Can you work these out from the model? Positions are in its coordinate system, mm. A direction names the side the tool comes from. Coordinates: 2 decimals unless noted, no trailing zeros. Loops run counter-clockwise (first coordinate to the right, second up) from the corner with the lowest first, then second, coordinate; pieces in that order, holes last.
```python
from build123d import *

# Parameters (mm, degrees)
BOSS_EXTRUDE1_DEPTH = 9
SKETCH2_R           = 1.2
CUT_EXTRUDE1_DEPTH  = 29


with BuildPart() as part:
    # Sketch1 → Boss-Extrude1 (new body)
    with BuildSketch(Plane.XY):
        Polygon((7.5, 1), (7.5, 11.5), (-7.5, 11.5), (-7.5, 1), (-11.5, 1), (-11.5, 0), (-6.5, 0), (-6.5, 10.5), (6.5, 10.5), (6.5, 0), (11.5, 0), (11.5, 1), align=None)
    extrude(amount=BOSS_EXTRUDE1_DEPTH)

    # Sketch2 → Cut-Extrude1 (cut)
    with BuildSketch(Plane(origin=(0, 1, 0), x_dir=(1, 0, 0), z_dir=(0, 1, 0))):
        with Locations((9.5, -4.5)):
            Circle(SKETCH2_R)
    cut_extrude1 = extrude(amount=-CUT_EXTRUDE1_DEPTH, mode=Mode.SUBTRACT)

    # Mirror1: Cut-Extrude1 across plane
    add(cut_extrude1.mirror(Plane(origin=(0, 0, 0), x_dir=(0, 0, 1), z_dir=(1, 0, 0))), mode=Mode.SUBTRACT)


solid = part.part
```
Item 1: I'm going to push flat-ended pins straight in: P1, Ø3, axis at x = -10, z = 6.5, coming from the +Y side; P2, Ø3, axis at x = -1, z = 7, coming from the -Y side; P3, Ø2.5, axis at y = 2.5, z = 6, coming from the -X side. Where does each tip first touch, or does it pass through?
Results are:
P1: stops at y = 1
P2: stops at y = 10.5
P3: stops at x = -7.5
Item 2: On a 3-axis mill with a long thin cutter (end or side, diameter ignored), from which of +Z, -Z, +X, -X, +Y, -Y can I reach the whole of each face in a straight line? I mean faces 4 (the face through (7.5, 6, 4)), 5 (the face through (-8.3, 0.51, 4.45)), 6 (the face through (-8, 0, 4)), 7 (the face through (-6.5, 5, 4)), 8 (the face through (-11, 1, 4)). Say none if no direction works.
Results are:
face 4: +Z, -Z, +X, +Y
face 5: +Y, -Y
face 6: +Z, -Z, +X, -X, -Y
face 7: +Z, -Z, -Y
face 8: +Z, -Z, -X, +Y
Item 3: Suppose I cut it at A-A, the plane x = 9.5. Please give me the cut outline in (y, z), plus the area to 3 significant figures.
Results are:
outline: (0, 0) - (1, 0) - (1, 3.3) - (0, 3.3) - close; (0, 5.7) - (1, 5.7) - (1, 9) - (0, 9) - close
area: 6.60 mm2
Item 4: Suppose I cut it at B-B, the plane y = 2. Please give me the cut outline in (x, z).
Results are:
outline: (-7.5, 0) - (-6.5, 0) - (-6.5, 9) - (-7.5, 9) - close; (6.5, 0) - (7.5, 0) - (7.5, 9) - (6.5, 9) - close
Item 5: I need wall thicknesses on line 1 along X through (y, z) = (0.5, 4.5); line 2 along Z through (x, y) = (9.5, 0.4); line 3 along X through (y, z) = (9.75, 1.5). Which ranges of each line are inside material? Lowest first, please.
Results are:
line 1: x = -11.5 to -10.7, -8.3 to -6.5, 6.5 to 8.3, 10.7 to 11.5
line 2: z = 0 to 3.3, 5.7 to 9
line 3: x = -7.5 to -6.5, 6.5 to 7.5
Item 6: We'd pull the mould along Z, two halves only. Please class faces 1 (the face through (8.3, 0.51, 4.45)), 2 (the face through (-7.5, 6, 4)), 3 (the face through (-1, 11, 0)): +Z half, -Z half, draft (parallel to the pull), parting line (faces both ways), or undercut.
Results are:
face 1: undercut
face 2: draft
face 3: -Z half
Item 7: Suppose I cut it at C-C, the plane z = 3.75. Please give me the cut outline in (x, y), plus the area to 3 significant figures.
Results are:
outline: (-11.5, 0) - (-10.44, 0) - (-10.44, 1) - (-11.5, 1) - close; (-8.56, 0) - (-6.5, 0) - (-6.5, 10.5) - (6.5, 10.5) - (6.5, 0) - (8.56, 0) - (8.56, 1) - (7.5, 1) - (7.5, 11.5) - (-7.5, 11.5) - (-7.5, 1) - (-8.56, 1) - close; (10.44, 0) - (11.5, 0) - (11.5, 1) - (10.44, 1) - close
area: 40.3 mm2
Item 8: Suppose I cut it at D-D, the plane z = 2.25. Please give me the cut outline in (x, y), plus the area to 3 significant figures.
Results are:
outline: (-11.5, 0) - (-6.5, 0) - (-6.5, 10.5) - (6.5, 10.5) - (6.5, 0) - (11.5, 0) - (11.5, 1) - (7.5, 1) - (7.5, 11.5) - (-7.5, 11.5) - (-7.5, 1) - (-11.5, 1) - close
area: 44.0 mm2
